from build123d import *

# Parameters (mm, degrees)
SKETCH1_W           = 7.62
SKETCH1_H           = 33.02
SKETCH1_R           = 2.12725
BOSS_EXTRUDE1_DEPTH = 50.8


with BuildPart() as part:
    # Sketch1 → Boss-Extrude1 (new, symmetric)
    with BuildSketch(Plane(origin=(0, 0, 0), x_dir=(1, 0, 0), z_dir=(0, 1, 0))):
        with Locations((-142.038308124, -19.2875)):
            Rectangle(SKETCH1_W, SKETCH1_H)
        with Locations(Location((-142.038308124, -6.5875, 0), (0, 0, 270))):
            Circle(SKETCH1_R, mode=Mode.SUBTRACT)
        with Locations(Location((-142.038308124, -31.9875, 0), (0, 0, 270))):
            Circle(SKETCH1_R, mode=Mode.SUBTRACT)
    extrude(amount=BOSS_EXTRUDE1_DEPTH, both=True)


solid = part.part
Verification items for the finished model (mm, model axes). Round coordinates to 2 decimals unless told otherwise and drop trailing zeros. Loops run counter-clockwise (first coordinate to the right, second up) from the corner with the lowest first, then second, coordinate; pieces in that order, holes last. Notation, with made-up numbers: (83, 62.5) - (128, 62.5) arc R19 ccw to (128, 96.5) - close; hole circle Ø10 at (79, 78.25). An arc over 180 degrees is marked (long way). Use one line per item in the form item = value.
1. Section check A-A on z = 33. Record the cut outline in (x, y), and give its area (3 significant figures).
A:
outline = (-145.85, -50.8) - (-143.91, -50.8) - (-143.91, 50.8) - (-145.85, 50.8) - close; (-140.17, -50.8) - (-138.23, -50.8) - (-138.23, 50.8) - (-140.17, 50.8) - close
area = 394 mm²
2. Draft check along Z on faces 1 (the flat face through (-142, 1, 2.778)), 2 (the flat face through (-138.228, 1, 20)), 3 (the cylindrical face through (-144.115, -0.711, 6.126)), 4 (the cylindrical face through (-144.115, -0.711, 31.526)). Enter one of: pulls with the +Z half, pulls with the -Z half, needs draft (parallel to the pull), parting line crosses it, or undercut.
A:
face_1 = pulls with the -Z half
face_2 = needs draft
face_3 = undercut
face_4 = undercut
3. Scan lines: probe 1 along Z at (x, y) = (-141.75, 30.5); probe 2 along Z at (x, y) = (-143.25, 19.5); probe 3 along X at (y, z) = (-23, 5). Record each from-to range of solid material in increasing order.
A:
probe_1 = 2.78 to 4.48, 8.7 to 29.88, 34.1 to 35.8
probe_2 = 2.78 to 4.84, 8.34 to 30.24, 33.74 to 35.8
probe_3 = -145.85 to -143.45, -140.62 to -138.23
4. Section check C-C on y = 20. Record the cut outline in (x, z), and give its area (3 significant figures).
A:
outline = (-145.85, 2.78) - (-138.23, 2.78) - (-138.23, 35.8) - (-145.85, 35.8) - close; hole circle Ø4.25 at (-142.04, 6.59); hole circle Ø4.25 at (-142.04, 31.99)
area = 223 mm²
5. Section check B-B on x = -143. Record the cut outline in (y, z).
A:
outline = (-50.8, 2.78) - (50.8, 2.78) - (50.8, 4.69) - (-50.8, 4.69) - close; (-50.8, 8.48) - (50.8, 8.48) - (50.8, 30.09) - (-50.8, 30.09) - close; (-50.8, 33.88) - (50.8, 33.88) - (50.8, 35.8) - (-50.8, 35.8) - close
6. Gauge pin test, flat end, axial feed: pin 1 Ø3.5 at (x, z) = (-142.04, 31.99) entering from -Y. Record the tip position at first contact, or that the pin passes through.
A:
pin_1 = through
